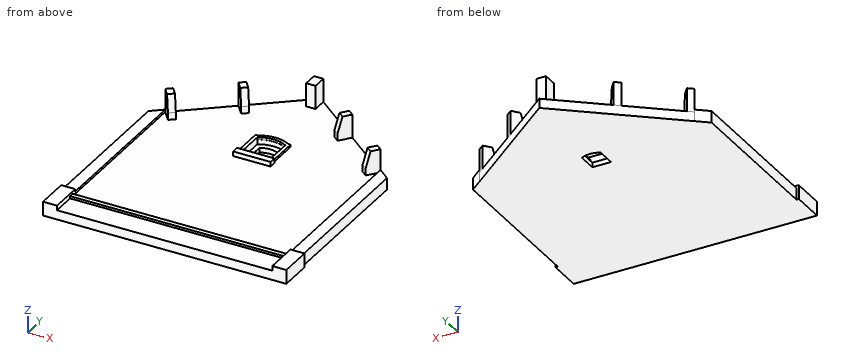
```python
from build123d import *

# Parameters (mm, degrees)
PAD_DEPTH       = 2
POCKET_DEPTH    = 1
POCKET001_DEPTH = 5
SKETCH003_W     = 8
SKETCH003_H     = 1.5
PAD001_DEPTH    = 1
SKETCH006_W     = 3
SKETCH006_H     = 7
PAD004_DEPTH    = 3
PAD005_DEPTH    = 2.5
SKETCH008_W     = 46
SKETCH008_H     = 1
PAD006_DEPTH    = 0.5
PAD008_DEPTH    = 0.5
SKETCH013_W     = 2
SKETCH013_H     = 3.0000000001
PAD009_DEPTH    = 5
POCKET002_DEPTH = 20
POCKET003_DEPTH = 20


with BuildPart() as part:
    # Sketch → Pad (new body)
    with BuildSketch(Plane.XY):
        Polygon((-25, -20), (25, -20), (25, 20), (0, 40), (-25, 20), align=None)
    extrude(amount=PAD_DEPTH)

    # Sketch001 → Pocket (cut)
    with BuildSketch(Plane.XY.offset(2)):
        with BuildLine():
            Line((-3, 15), (3, 15))
            Line((3, 15), (3, 21))
            ThreePointArc((3, 21), (0, 21.8038475773), (-3, 21))
            Line((-3, 15), (-3, 21))
        make_face()
    extrude(amount=-POCKET_DEPTH, mode=Mode.SUBTRACT)

    # Sketch002 → Pocket001 (cut)
    with BuildSketch(Plane.XY.offset(1)):
        with BuildLine():
            Line((-2, 16), (2, 16))
            Line((2, 16), (2, 20))
            ThreePointArc((2, 20), (0, 20.5358983849), (-2, 20))
            Line((-2, 16), (-2, 20))
        make_face()
    extrude(amount=-POCKET001_DEPTH, mode=Mode.SUBTRACT)

    # Sketch003 → Pad001 (new body)
    with BuildSketch(Plane.XY.offset(2)):
        with Locations((0, 14.25)):
            Rectangle(SKETCH003_W, SKETCH003_H)
    extrude(amount=PAD001_DEPTH)

    # Sketch006 → Pad004 (new body)
    with BuildSketch(Plane(origin=(0, 0, 0), x_dir=(1, 0, 0), z_dir=(0, 0, -1))):
        with Locations((-24.5, 16.5)):
            Rectangle(SKETCH006_W, SKETCH006_H)
        with Locations((24.5, 16.5)):
            Rectangle(SKETCH006_W, SKETCH006_H)
    extrude(amount=-PAD004_DEPTH)

    # Sketch007 → Pad005 (new body)
    with BuildSketch(Plane(origin=(0, 0, 0), x_dir=(1, 0, 0), z_dir=(0, 0, -1))):
        Polygon((-25.5, 20), (-23, 20), (-23, -21.624460083), (-25.5, -19.6), align=None)
        Polygon((23, 20), (25.5, 20), (25.5, -19.6), (23, -21.624460083), align=None)
    extrude(amount=-PAD005_DEPTH)

    # Sketch008 → Pad006 (new body)
    with BuildSketch(Plane.XY.offset(2)):
        with Locations((0, -14.5)):
            Rectangle(SKETCH008_W, SKETCH008_H)
    extrude(amount=PAD006_DEPTH)

    # Sketch012 → Pad008 (new body)
    with BuildSketch(Plane.XY.offset(2)):
        with BuildLine():
            Line((3.3030993045, 21.6561501911), (3.75, 21.6561501911))
            Line((3.75, 21.6561501911), (3.75, 15))
            Line((3.75, 15), (3, 15))
            Line((3, 15), (3, 21))
            ThreePointArc((3, 21), (0, 21.8309518948), (-3, 21))
            Line((-3, 21), (-3, 15))
            Line((-3, 15), (-3.75, 15))
            Line((-3.75, 15), (-3.75, 21.6561501911))
            Line((-3.75, 21.6561501911), (-3.3030993046, 21.6561501911))
            ThreePointArc((-3.3030993046, 21.6561501911), (0, 22.55), (3.3030993045, 21.6561501911))
        make_face()
    extrude(amount=PAD008_DEPTH)

    # Sketch013 → Pad009 (new body)
    with BuildSketch(Plane.XY.offset(2)):
        Polygon((-23, 21.6), (-21.1259148573, 19.2573935717), (-19.9546116432, 20.194436143), (-21.8286967858, 22.5370425713), align=None)
        Polygon((-12.1713032142, 30.2629574287), (-11, 31.2), (-9.1259148573, 28.8573935717), (-10.2972180715, 27.9203510003), align=None)
        with Locations((0, 37.7)):
            Rectangle(SKETCH013_W, SKETCH013_H)
        Polygon((11, 31.2), (12.1713032142, 30.2629574287), (10.2972180715, 27.9203510003), (9.1259148573, 28.8573935717), align=None)
        Polygon((21.8286967858, 22.5370425713), (23, 21.6), (21.1259148573, 19.2573935717), (19.9546116432, 20.194436143), align=None)
    extrude(amount=PAD009_DEPTH)

    # Sketch014 → Pocket002 (cut)
    with BuildSketch(Plane(origin=(-3.487804878, -2.7902439024, 0), x_dir=(0.6246950476, -0.7808688094, 0), z_dir=(-0.7808688094, -0.6246950476, 0))):
        Polygon((-29.2347523777, 7), (-28.2347523777, 7), (-28.2347523777, 3.5), align=None)
    extrude(amount=-POCKET002_DEPTH, mode=Mode.SUBTRACT)

    # Sketch015 → Pocket003 (cut)
    with BuildSketch(Plane(origin=(3.487804878, -2.7902439024, 0), x_dir=(0.6246950476, 0.7808688094, 0), z_dir=(0.7808688094, -0.6246950476, 0))):
        Polygon((29.2347523777, 7), (28.2347523777, 7), (28.2347523777, 3.5), align=None)
    extrude(amount=-POCKET003_DEPTH, mode=Mode.SUBTRACT)


solid = part.part
```
The model under review builds one solid part; all positions refer to its coordinate system, in mm. Round coordinates to 2 decimals unless told otherwise and drop trailing zeros. Order: outer loops, then holes, each group sorted by start corner. A loop starts at its lowest first (then second) coordinate and runs counter-clockwise, first axis right, second up.
(1) Take a section at D-D, the plane y = 6.5. State the section outline as (x, z) points, plus the area to 4 significant figures.
Working result:
outline: (-25.5, 0) - (25.5, 0) - (25.5, 2.5) - (23, 2.5) - (23, 2) - (-23, 2) - (-23, 2.5) - (-25.5, 2.5) - close
area: 104.5 mm2
(2) Take a section at C-C, the plane x = -16. State the section outline as (y, z) points.
Working result:
outline: (-20, 0) - (27.2, 0) - (27.2, 2) - (-14, 2) - (-14, 2.5) - (-15, 2.5) - (-15, 2) - (-20, 2) - close
(3) Wall thickness on L1, parallel to X at y = 22, z = 2.25; L2, parallel to Z at x = 11, y = 25; L3, parallel to X at y = 21.5, z = 4.5: over which ranges is each line inside the solid? List them lowest first.
Working result:
L1: x = -22.5 to -21.4, -2.63 to 2.63, 21.4 to 22.5
L2: z = 0 to 2
L3: x = -22.92 to -21, 21 to 22.92
(4) Take a section at A-A, the plane y = 18. State the section outline as (x, z) points, plus the area to 4 significant figures.
Working result:
outline: (-25.5, 0) - (-2, 0) - (-2, 1) - (-3, 1) - (-3, 2.5) - (-3.75, 2.5) - (-3.75, 2) - (-23, 2) - (-23, 2.5) - (-25.5, 2.5) - close; (2, 0) - (25.5, 0) - (25.5, 2.5) - (23, 2.5) - (23, 2) - (3.75, 2) - (3.75, 2.5) - (3, 2.5) - (3, 1) - (2, 1) - close
area: 95.25 mm2
(5) Take a section at B-B, the plane z = 5.5. State the section outline as (x, y) points.
Working result:
outline: (-23, 21.6) - (-21.48, 19.7) - (-20.31, 20.64) - (-21.83, 22.54) - close; (-12.17, 30.26) - (-10.65, 28.37) - (-9.48, 29.3) - (-11, 31.2) - close; (-1, 36.2) - (1, 36.2) - (1, 39.2) - (-1, 39.2) - close; (9.48, 29.3) - (10.65, 28.37) - (12.17, 30.26) - (11, 31.2) - close; (20.31, 20.64) - (21.48, 19.7) - (23, 21.6) - (21.83, 22.54) - close
(6) For P1, Ø1.5, axis at x = -17.5, y = -12.5, coming from the -Z side; P2, Ø3, axis at x = 24.5, y = -1.5, coming from the +Z side; P3, Ø0.8, axis at y = 17.5, z = 0.5, coming from the +X side; P4, Ø0.6, axis at x = -1.5, z = 2.5, coming from the -Y side, all flat-tipped, find the tip position at first contact; note any pin that passes through.
Working result:
P1: stops at z = 0
P2: stops at z = 2.5
P3: stops at x = 25.5
P4: stops at y = -15
